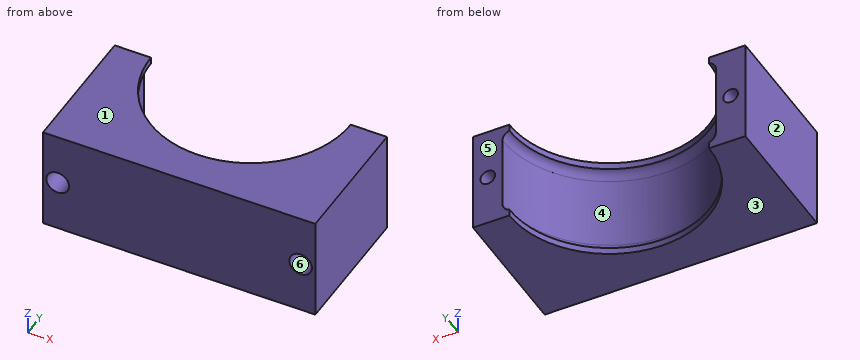
Autodesk Inventor part; units mm, degrees
ref_plane "YZ Plane" through (0, 0, 0) normal (1, 0, 0) x (0, 1, 0)
ref_plane "XZ Plane" through (0, 0, 0) normal (0, 1, 0) x (-1, 0, 0)
ref_plane "XY Plane" through (0, 0, 0) normal (0, 0, 1) x (1, 0, 0)
sketch "Sketch1" plane through (0, 0, 0) normal (0, 0, 1) x (1, 0, 0)
  arc A0 (-23.5, 0) -> (23.5, 0) centre (0, 0) ccw
  line L0 (30, 0) -> (30, -30)
  line L1 (30, -30) -> (-30, -30)
  line L2 (-30, -30) -> (-30, 0)
  line L3 (-30, 0) -> (-23.5, 0)
  line L4 (23.5, 0) -> (30, 0)
  dimension "d0" = 47
  dimension "d1" = 30
  dimension "d3" = 60
  dimension "d4" = 30
extrude "Extrusion1" add sketch "Sketch1" along normal blind 23
ref_plane "Work Plane1" through (0, 0, 23) normal (0, 0, 1) x (1, 0, 0)
sketch "Sketch2" plane through (0, 0, 23) normal (0, 0, 1) x (1, 0, 0)
  line L0 (30, 0) -> (23.5, 0)
  arc A0 (-23.5, 0) -> (23.5, 0) centre (0, 0) ccw
  arc A1 (-22, 0) -> (22, 0) centre (0, 0) ccw
  line L1 (-23.5, 0) -> (-22, 0)
  line L2 (22, 0) -> (23.5, 0)
  dimension "d8" = 44
extrude "Extrusion2" add sketch "Sketch2" against normal blind 1.5
fillet "Fillet1" radius 2 1 edges at (0, -23.5, 21.5)
ref_plane "Work Plane2" through (0, 0, 0) normal (0, 0, -1) x (-1, 0, 0)
sketch "Sketch3" plane through (0, 0, 0) normal (0, 0, -1) x (-1, 0, 0)
  arc A0 (-23.5, 0) -> (23.5, 0) centre (0, 0) ccw
  arc A1 (-22, 0) -> (22, 0) centre (0, 0) ccw
  line L0 (23.5, 0) -> (30, 0)
  line L1 (23.5, 0) -> (22, 0)
  line L2 (-22, 0) -> (-23.5, 0)
extrude "Extrusion3" add sketch "Sketch3" against normal blind 1.5
fillet "Fillet2" radius 2 1 edges at (0, -23.5, 1.5)
sketch "Sketch4" plane through (-30, 0, 23) normal (0, 1, 0) x (1, 0, 0)
  line L0 (-12, 23) -> (72, 23)
  line L1 (0, 23) -> (0, 0)
  line L2 (53.5, 19.5635) -> (53.5, 3.4365)
  point P0 (30, 23)
  point P1 (3.25, 11.5)
  point P2 (56.75, 11.5)
  dimension "d16" = 11.5
  dimension "d17" = 3.25
  dimension "d18" = 3.25
hole "Hole1" at (-26.75, 0, 11.5) at (26.75, 0, 11.5) direction (0, -1, 0) diameter 3.242 end through all
sketch "Sketch5" plane through (-30, -30, 0) normal (0, -1, 0) x (1, 0, 0)
  line L0 (0, 0) -> (0, 23)
  line L1 (0, 0) -> (60, 0)
  circle A0 centre (3.25, 11.5) radius 2.5
  circle A1 centre (56.75, 11.5) radius 1.621
  circle A2 centre (56.75, 11.5) radius 2.5
  point P0 (30, 0)
  dimension "d26" = 3.25
  dimension "d27" = 11.5
  dimension "d28" = 5
  dimension "d29" = 5
extrude "Extrusion4" cut sketch "Sketch5" against normal blind 6
equation "\"d24\" = Thickness"
equation "\"BendRadius\" = Thickness"
equation "\"BendReliefWidth\" = Thickness"
equation "\"BendReliefDepth\" = 0.5 * Thickness"
equation "\"CornerReliefSize\" = 4 * Thickness"
equation "\"MinimumRemnant\" = 2 * Thickness"
equation "\"TransitionRadius\" = BendRadius"
equation "\"JacobiRadiusSize\" = BendRadius"
equation "\"GapSize\" = Thickness"
properties part number "Bearing housing top"
Here's how the part is built. I have some questions about the finished solid (model axes, mm). Face numbers are marked on the shaded views. A direction names the side the tool comes from. Give positions to 0.01 mm unless a question says otherwise; leave off trailing zeros. Order: outer loops, then holes, each group sorted by start corner. A loop starts at its lowest first (then second) coordinate and runs counter-clockwise, first axis right, second up. Notation, with made-up numbers: M -11,83 L 35,83 A16 ccw 35,105 Z; hole C 52,58.25 d2. An arc over 180 degrees is marked long. Answer as a JSON object with one key per item and string values. Group by question number.
1) Suppose I cut it at D-D, the plane z = 17.25. Write out the boundary of the cut face in (x, y).
2) We'd pull the mould along Z, two halves only. Please class the marked faces 1, 2, 3 and 4: pulls with the +Z half, pulls with the -Z half, needs draft (parallel to the pull), parting line crosses it, or undercut.
3) Suppose I cut it at A-A, the plane z = 11.5. Write out the boundary of the cut face in (x, y).
4) Suppose I cut it at B-B, the plane x = 26.75. Write out the boundary of the cut face in (y, z).
5) Suppose I cut it at C-C, the plane x = 0. Write out the boundary of the cut face in (y, z), plus the area to 3 significant figures.
6) Please list where these lines run through material, in increasing order: L1, parallel to Z at x = 26.75, y = -25.65; L2, parallel to Z at x = 17, y = -14; L3, parallel to X at y = -27.25, z = 13.5. Write a range as [from, to].
7) On a 3-axis mill with a long thin cutter (end or side, diameter ignored), from which of +Z, -Z, +X, -X, +Y, -Y can I reach the whole of each face in a straight line? I mean the marked faces 5 and 6. Say none if no direction works.
8) I'm going to push flat-ended pins straight in: pin 1 Ø4.5 at (x, z) = (-26.75, 11.5) entering from -Y; pin 2 Ø1.5 at (x, z) = (-18, 8) entering from +Y. Where does each tip first touch, or does it pass through?
Results found:
{
 "1": {"outline": "M -30,-30 L 30,-30 L 30,0 L 23.5,0 A23.5 cw -23.5,0 L -30,0 Z"},
 "2": {"face 1": "pulls with the +Z half", "face 2": "needs draft", "face 3": "pulls with the -Z half", "face 4": "undercut"},
 "3": {"outline": "M -30,-30 L -29.25,-30 L -29.25,-24 L -28.37,-24 L -28.37,0 L -30,0 Z; M -25.13,-24 L -24.25,-24 L -24.25,-30 L 24.25,-30 L 24.25,-24 L 25.13,-24 L 25.13,0 L 23.5,0 A23.5 cw -23.5,0 L -25.13,0 Z; M 28.37,-24 L 29.25,-24 L 29.25,-30 L 30,-30 L 30,0 L 28.37,0 Z"},
 "4": {"outline": "M -30,0 L 0,0 L 0,9.88 L -24,9.88 L -24,9 L -30,9 Z; M -30,14 L -24,14 L -24,13.12 L 0,13.12 L 0,23 L -30,23 Z"},
 "5": {"outline": "M -30,0 L -22,0 L -22,1.5 A2 cw -23.5,3.44 L -23.5,19.56 A2 cw -22,21.5 L -22,23 L -30,23 Z", "area": "156 mm²"},
 "6": {"L1": "[0, 9], [14, 23]", "L2": "[0, 1.51], [21.49, 23]", "L3": "[-30, -28.25], [-25.25, 25.25], [28.25, 30]"},
 "7": {"face 5": "+Z, -Z, +X, -X, +Y", "face 6": "-Y"},
 "8": {"pin 1": "y = -24", "pin 2": "y = -14.17"}
}
